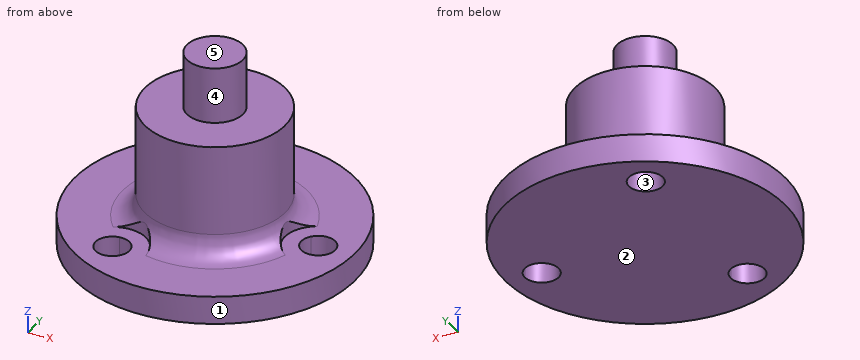
```python
from build123d import *

# Parameters (mm, degrees)
F3_DEPTH = 12.7
F4_DEPTH = 24.001


with BuildPart() as f1:
    # F0 (on Front) → F1 (revolve)
    with BuildSketch(Plane.XZ):
        with BuildLine():
            Line((0, 28), (0, 0))
            Line((0, 0), (20, 0))
            Line((20, 0), (20, 4))
            Line((20, 4), (13.175, 4))
            ThreePointArc((13.175, 4), (10.9299359697, 4.9299359697), (10, 7.175))
            Line((10, 7.175), (10, 20))
            Line((10, 20), (4, 20))
            Line((4, 20), (4, 28))
            Line((4, 28), (0, 28))
        make_face()
    revolve(axis=Axis((0, 0, 14), (0, 0, -1)))

    # F2 (on face) → F3 (cut, symmetric)
    with BuildSketch(Plane.XY.offset(4)):
        with BuildLine():
            ThreePointArc((-7.8251834884, 10.5993928304), (-6.2935, 10.9006617574), (-5.2667517116, 12.0765041054))
            ThreePointArc((-5.2667517116, 12.0765041054), (-6.5875, 11.4098846949), (-7.8251834884, 10.5993928304))
        make_face()
        with BuildLine():
            ThreePointArc((-7.8251834884, 10.5993928304), (-6.5875, 11.4098846949), (-5.2667517116, 12.0765041054))
            ThreePointArc((-5.2667517116, 12.0765041054), (-5.1323643524, 12.5246875524), (-5.087, 12.9903810568))
            ThreePointArc((-5.087, 12.9903810568), (-9.087120229, 14.8079669224), (-7.8251834884, 10.5993928304))
        make_face()
        with BuildLine():
            ThreePointArc((13.0919352, -1.4771112751), (15.7805154187, -2.2832793699), (17.413, 0))
            ThreePointArc((17.413, 0), (15.7805154187, 2.2832793699), (13.0919352, 1.4771112751))
            ThreePointArc((13.0919352, 1.4771112751), (13.1542174085, 0.7397224953), (13.175, 0))
            ThreePointArc((13.175, 0), (13.1542174085, -0.7397224953), (13.0919352, -1.4771112751))
        make_face()
        with BuildLine():
            ThreePointArc((13.175, 0), (13.1542174085, 0.7397224953), (13.0919352, 1.4771112751))
            ThreePointArc((13.0919352, 1.4771112751), (12.587, 0), (13.0919352, -1.4771112751))
            ThreePointArc((13.0919352, -1.4771112751), (13.1542174085, -0.7397224953), (13.175, 0))
        make_face()
        with BuildLine():
            ThreePointArc((-7.8251834884, -10.5993928304), (-6.5875, -11.4098846949), (-5.2667517116, -12.0765041054))
            ThreePointArc((-5.2667517116, -12.0765041054), (-6.2935, -10.9006617574), (-7.8251834884, -10.5993928304))
        make_face()
        with BuildLine():
            ThreePointArc((-5.087, -12.9903810568), (-5.1323643524, -12.5246875524), (-5.2667517116, -12.0765041054))
            ThreePointArc((-5.2667517116, -12.0765041054), (-6.5875, -11.4098846949), (-7.8251834884, -10.5993928304))
            ThreePointArc((-7.8251834884, -10.5993928304), (-9.087120229, -14.8079669224), (-5.087, -12.9903810568))
        make_face()
    extrude(amount=F3_DEPTH, both=True, mode=Mode.SUBTRACT)

    # F2 (on face) → F4 (cut, through all)
    with BuildSketch(Plane.XY.offset(4)):
        with BuildLine():
            ThreePointArc((-5.2667517116, 12.0765041054), (-4.0231580631, 12.545709394), (-2.7386172875, 12.8872262474))
            ThreePointArc((-2.7386172875, 12.8872262474), (-2.7377793301, 12.9388006268), (-2.7375, 12.9903810568))
            ThreePointArc((-2.7375, 12.9903810568), (-9.9257802977, 17.0887949204), (-9.7913566709, 8.8153252659))
            ThreePointArc((-9.7913566709, 8.8153252659), (-8.8533240122, 9.7570117831), (-7.8251834884, 10.5993928304))
            ThreePointArc((-7.8251834884, 10.5993928304), (-9.087120229, 14.8079669224), (-5.087, 12.9903810568))
            ThreePointArc((-5.087, 12.9903810568), (-5.1323643524, 12.5246875524), (-5.2667517116, 12.0765041054))
        make_face()
        with BuildLine():
            ThreePointArc((-9.7913566709, 8.8153252659), (-5.11875, 8.8659350712), (-2.7386172875, 12.8872262474))
            ThreePointArc((-2.7386172875, 12.8872262474), (-4.0231580631, 12.545709394), (-5.2667517116, 12.0765041054))
            ThreePointArc((-5.2667517116, 12.0765041054), (-6.2935, 10.9006617574), (-7.8251834884, 10.5993928304))
            ThreePointArc((-7.8251834884, 10.5993928304), (-8.8533240122, 9.7570117831), (-9.7913566709, 8.8153252659))
        make_face()
        with BuildLine():
            ThreePointArc((13.0919352, -1.4771112751), (12.587, 0), (13.0919352, 1.4771112751))
            ThreePointArc((13.0919352, 1.4771112751), (12.8764820753, 2.788697611), (12.5299739583, 4.0719009815))
            ThreePointArc((12.5299739583, 4.0719009815), (10.2375, 0), (12.5299739583, -4.0719009815))
            ThreePointArc((12.5299739583, -4.0719009815), (12.8764820753, -2.788697611), (13.0919352, -1.4771112751))
        make_face()
        with BuildLine():
            ThreePointArc((13.0919352, 1.4771112751), (15.7805154187, 2.2832793699), (17.413, 0))
            ThreePointArc((17.413, 0), (15.7805154187, -2.2832793699), (13.0919352, -1.4771112751))
            ThreePointArc((13.0919352, -1.4771112751), (12.8764820753, -2.788697611), (12.5299739583, -4.0719009815))
            ThreePointArc((12.5299739583, -4.0719009815), (17.3364403723, -4.1499942936), (19.7625, 0))
            ThreePointArc((19.7625, 0), (17.3364403723, 4.1499942936), (12.5299739583, 4.0719009815))
            ThreePointArc((12.5299739583, 4.0719009815), (12.8764820753, 2.788697611), (13.0919352, 1.4771112751))
        make_face()
        with BuildLine():
            ThreePointArc((-5.2667517116, -12.0765041054), (-4.0231580631, -12.545709394), (-2.7386172875, -12.8872262474))
            ThreePointArc((-2.7386172875, -12.8872262474), (-5.11875, -8.8659350712), (-9.7913566709, -8.8153252659))
            ThreePointArc((-9.7913566709, -8.8153252659), (-8.8533240122, -9.7570117831), (-7.8251834884, -10.5993928304))
            ThreePointArc((-7.8251834884, -10.5993928304), (-6.2935, -10.9006617574), (-5.2667517116, -12.0765041054))
        make_face()
        with BuildLine():
            ThreePointArc((-2.7375, -12.9903810568), (-2.7377793301, -12.9388006268), (-2.7386172875, -12.8872262474))
            ThreePointArc((-2.7386172875, -12.8872262474), (-4.0231580631, -12.545709394), (-5.2667517116, -12.0765041054))
            ThreePointArc((-5.2667517116, -12.0765041054), (-5.1323643524, -12.5246875524), (-5.087, -12.9903810568))
            ThreePointArc((-5.087, -12.9903810568), (-9.087120229, -14.8079669224), (-7.8251834884, -10.5993928304))
            ThreePointArc((-7.8251834884, -10.5993928304), (-8.8533240122, -9.7570117831), (-9.7913566709, -8.8153252659))
            ThreePointArc((-9.7913566709, -8.8153252659), (-9.9257802977, -17.0887949204), (-2.7375, -12.9903810568))
        make_face()
    extrude(amount=F4_DEPTH, mode=Mode.SUBTRACT)


solid = f1.part
```
The model under review builds one solid part; all positions refer to its coordinate system, in mm. Face numbers are marked on the shaded views. A direction names the side the tool comes from. Coordinates: 2 decimals unless noted, no trailing zeros. Order: outer loops, then holes, each group sorted by start corner. A loop starts at its lowest first (then second) coordinate and runs counter-clockwise, first axis right, second up. Notation, with made-up numbers: (62.5, -7) -> (88.5, -7) arc R12 cw to (88.5, -1) -> close; hole circle Ø11 at (36.25, -34). An arc over 180 degrees is marked (long way). Answer in a Markdown table with one row per item. Add a question column.
Item 1: We need section B-B on x = 16.5. Write out the cut boundary in (y, z).
Item 2: We need section A-A on y = 14.5. Write out the cut boundary in (x, z), plus the area to 3 significant figures.
Item 3: Clearance check with flat-ended pins moving along their axes: pin 1 (3 mm diameter, centred on x = 8, y = 0, fed in from -Z); pin 2 (4 mm diameter, centred on x = -7.5, y = 12.99, fed in from +Z); pin 3 (5 mm diameter, centred on x = -3, z = 17, fed in from +Y); pin 4 (5 mm diameter, centred on x = -7, z = 3.5, fed in from +Y). State where each tip first meets the part, or that it passes through.
Item 4: We need section D-D on x = 0. Write out the cut boundary in (y, z) (3 decimals), plus the area to 3 significant figures.
Item 5: Machinability: for the marked faces 4 and 5, which of the approach directions +Z, -Z, +X, -X, +Y, -Y give a long, thin tool a straight path to every point of the face, cutting with its end or side? Answer none if there is none.
Item 6: We need section C-C on z = 2.5. Write out the cut boundary in (x, y).
Item 7: Mouldability with a two-part tool opening along Y and no side actions: class the marked faces 1, 2 and 3 as +Y half, -Y half, draft (parallel to the pull), parting line (faces both ways), or undercut.
Item 8: To check wall thickness, follow probe 1 along Y at (x, z) = (-7.5, 2.8); probe 2 along Z at (x, y) = (-15, -7); probe 3 along X at (y, z) = (0, 21.75). State the ranges of each line that lie inside material, in increasing order.
Final values:
| question | item | result |
|---|---|---|
| 1 | outline | (-11.3, 0) -> (-1.89, 0) -> (-1.89, 4) -> (-11.3, 4) -> close; (1.89, 0) -> (11.3, 0) -> (11.3, 4) -> (1.89, 4) -> close |
| 2 | outline | (-13.77, 0) -> (-9.38, 0) -> (-9.38, 4) -> (-13.77, 4) -> close; (-5.62, 0) -> (13.77, 0) -> (13.77, 4) -> (-5.62, 4) -> close |
| 2 | area | 95.1 mm2 |
| 3 | pin 1 | stops at z = 0 |
| 3 | pin 2 | passes through |
| 3 | pin 3 | stops at y = 9.99 |
| 3 | pin 4 | stops at y = 19.49 |
| 4 | outline | (-20, 0) -> (20, 0) -> (20, 4) -> (13.175, 4) arc R3.175 cw to (10, 7.175) -> (10, 20) -> (4, 20) -> (4, 28) -> (-4, 28) -> (-4, 20) -> (-10, 20) -> (-10, 7.175) arc R3.175 cw to (-13.175, 4) -> (-20, 4) -> close |
| 4 | area | 548 mm2 |
| 5 | face 4 | +Z |
| 5 | face 5 | +Z, +X, -X, +Y, -Y |
| 6 | outline | circle Ø40 at (0, 0); hole circle Ø4.83 at (-7.5, -12.99); hole circle Ø4.83 at (-7.5, 12.99); hole circle Ø4.83 at (15, 0) |
| 7 | face 1 | parting line |
| 7 | face 2 | draft |
| 7 | face 3 | undercut |
| 8 | probe 1 | y = -18.54 to -15.4, -10.58 to 10.58, 15.4 to 18.54 |
| 8 | probe 2 | z = 0 to 4 |
| 8 | probe 3 | x = -4 to 4 |
